Could you check a few things on this model? Use its own coordinates, in mm. Face numbers are marked on the shaded views. A direction names the side the tool comes from. Give positions to 0.01 mm unless a question says otherwise; leave off trailing zeros. Loops run counter-clockwise (first coordinate to the right, second up) from the corner with the lowest first, then second, coordinate; pieces in that order, holes last.
1. Thinking about a two-plate mould opening in Z: for the marked faces 1, 2 and 3, which applies, +Z half, -Z half, draft (parallel to the pull), parting line (faces both ways), or undercut?
2. For the marked faces 4 and 5, which set-ups out of +Z, -Z, +X, -X, +Y, -Y let a thin tool reach every point of the face, with its end or its side?
3. Imagine slicing it at D-D (x = -113). List the corners of the cut face in (y, z) for me, plus the area to 3 significant figures.
4. Imagine slicing it at A-A (y = 39.5). List the corners of the cut face in (x, z) for me, plus the area to 3 significant figures.
5. I need wall thicknesses on line 1 along Z through (x, y) = (-99.5, 18); line 2 along X through (y, z) = (8, 0); line 3 along Z through (x, y) = (-61.5, 8.25). Which ranges of each line are inside material? Lowest first, please.
6. Imagine slicing it at B-B (x = -39). List the corners of the cut face in (y, z) for me, plus the area to 3 significant figures.
7. Imagine slicing it at C-C (y = 5). Count the separate pieces of the cut face and the enclosed holes in it, plus the area to 3 significant figures.
8. For P1, Ø1.5, axis at x = -52.5, z = 15, coming from the +Y side; P2, Ø3.5, axis at y = 18.5, z = -28, coming from the +X side; P3, Ø11, axis at x = -90, z = 0, coming from the -Y side (3 decimals); P4, Ø4, axis at y = 21, z = -11, coming from the -X side, each with a flat end and sliding along its axis, tell me the tip position at first contact or that it passes through.
```python
from build123d import *

# Parameters (mm, degrees)
BOSS_EXTRUDE1_DEPTH        = 10
BOSS_EXTRUDE2_DEPTH        = 32
CUT_EXTRUDE1_REACH         = 207
SKETCH3_R                  = 2.55
SKETCH3_W                  = 40
SKETCH3_H                  = 25
FILLET1_R                  = 1.2
SKETCH4_R                  = 7
SKETCH4_R_2                = 17.5
CUT_EXTRUDE2_DEPTH         = 11
SKETCH5_R                  = 21
CUT_EXTRUDE3_DEPTH         = 7
SKETCH6_R                  = 14
SKETCH6_R_2                = 11
BOSS_EXTRUDE3_DEPTH        = 6
CUT_EXTRUDE4_DEPTH         = 11
SKETCH8_R                  = 11
CUT_EXTRUDE5_DEPTH         = 7
SKETCH9_R                  = 2.1
SKETCH9_R_2                = 2.5
SKETCH9_R_3                = 1.6
CUT_EXTRUDE6_DEPTH         = 11
BOSS_EXTRUDE4_DEPTH        = 7
CHAMFER1_SIZE              = 2
LPATTERN1_COUNT            = 3
LPATTERN1_PITCH            = 40
CHAMFER1_OF_LPATTERN1_SIZE = 2
CUT_EXTRUDE7_DEPTH         = 12
LPATTERN2_COUNT            = 3
LPATTERN2_PITCH            = 64
MIRROR1_COPY_1_DEPTH       = 12
MIRROR1_COPY_2_DEPTH       = 12
CUT_REVOLVE1_ANGLE         = 20
SKETCH13_R                 = 11
CUT_EXTRUDE8_DEPTH         = 1


with BuildPart() as part:
    # Sketch1 → Boss-Extrude1 (new body)
    with BuildSketch(Plane(origin=(0, 0, 0), x_dir=(1, 0, 0), z_dir=(0, 1, 0))):
        with BuildLine():
            Line((0, 39), (-166, 39))
            Line((-166, 39), (-166, -39))
            Line((-166, -39), (0, -39))
            ThreePointArc((0, -39), (39, 0), (0, 39))
        make_face()
    extrude(amount=BOSS_EXTRUDE1_DEPTH)

    # Sketch2 → Boss-Extrude2 (add)
    with BuildSketch(Plane(origin=(0, 10, 0), x_dir=(1, 0, 0), z_dir=(0, 1, 0))):
        with BuildLine():
            Line((0, 39), (-166, 39))
            Line((-166, 39), (-166, -39))
            Line((-166, -39), (0, -39))
            ThreePointArc((0, -39), (39, 0), (0, 39))
        make_face()
        with BuildLine():
            Line((0, 35), (-158, 35))
            Line((-158, 35), (-158, -35))
            Line((-158, -35), (0, -35))
            ThreePointArc((0, -35), (35, 0), (0, 35))
        make_face(mode=Mode.SUBTRACT)
    extrude(amount=BOSS_EXTRUDE2_DEPTH)

    # Sketch3 → Cut-Extrude1 (cut, up to next)
    with BuildSketch(Plane.ZY.offset(166), mode=Mode.PRIVATE) as cut_extrude1_sk1:
        with Locations((-25.5, 34.5)):
            Circle(SKETCH3_R)
    cut_extrude1_tool1 = extrude(cut_extrude1_sk1.sketch, amount=-CUT_EXTRUDE1_REACH, mode=Mode.PRIVATE) & part.part
    add(cut_extrude1_tool1.solids().sort_by_distance((-166, 34.5, -25.5))[0], mode=Mode.SUBTRACT)
    # Sketch3 → Cut-Extrude1 (cut, up to next)
    with BuildSketch(Plane.ZY.offset(166), mode=Mode.PRIVATE) as cut_extrude1_sk2:
        with Locations((-25.5, 16.5)):
            Circle(SKETCH3_R)
    cut_extrude1_tool2 = extrude(cut_extrude1_sk2.sketch, amount=-CUT_EXTRUDE1_REACH, mode=Mode.PRIVATE) & part.part
    add(cut_extrude1_tool2.solids().sort_by_distance((-166, 16.5, -25.5))[0], mode=Mode.SUBTRACT)
    # Sketch3 → Cut-Extrude1 (cut, up to next)
    with BuildSketch(Plane.ZY.offset(166), mode=Mode.PRIVATE) as cut_extrude1_sk3:
        with Locations((25.5, 16.5)):
            Circle(SKETCH3_R)
    cut_extrude1_tool3 = extrude(cut_extrude1_sk3.sketch, amount=-CUT_EXTRUDE1_REACH, mode=Mode.PRIVATE) & part.part
    add(cut_extrude1_tool3.solids().sort_by_distance((-166, 16.5, 25.5))[0], mode=Mode.SUBTRACT)
    # Sketch3 → Cut-Extrude1 (cut, up to next)
    with BuildSketch(Plane.ZY.offset(166), mode=Mode.PRIVATE) as cut_extrude1_sk4:
        with Locations((25.5, 34.5)):
            Circle(SKETCH3_R)
    cut_extrude1_tool4 = extrude(cut_extrude1_sk4.sketch, amount=-CUT_EXTRUDE1_REACH, mode=Mode.PRIVATE) & part.part
    add(cut_extrude1_tool4.solids().sort_by_distance((-166, 34.5, 25.5))[0], mode=Mode.SUBTRACT)
    # Sketch3 → Cut-Extrude1 (cut, up to next)
    with BuildSketch(Plane.ZY.offset(166), mode=Mode.PRIVATE) as cut_extrude1_sk5:
        with Locations((0, 24.5)):
            Rectangle(SKETCH3_W, SKETCH3_H)
    cut_extrude1_tool5 = extrude(cut_extrude1_sk5.sketch, amount=-CUT_EXTRUDE1_REACH, mode=Mode.PRIVATE) & part.part
    add(cut_extrude1_tool5.solids().sort_by_distance((-166, 24.5, 0))[0], mode=Mode.SUBTRACT)

    # Fillet1
    fillet1_edges = [part.edges().sort_by_distance(p)[0] for p in [
        (-162, 37, -20),
        (-162, 12, -20),
        (-162, 12, 20),
        (-162, 37, 20),
    ]]
    fillet(fillet1_edges, radius=FILLET1_R)

    # Sketch4 → Cut-Extrude2 (cut, through all)
    with BuildSketch(Plane(origin=(0, 10, 0), x_dir=(1, 0, 0), z_dir=(0, 1, 0))):
        with Locations((-90, 0)):
            Circle(SKETCH4_R)
        Circle(SKETCH4_R_2)
    extrude(amount=-CUT_EXTRUDE2_DEPTH, mode=Mode.SUBTRACT)

    # Sketch5 → Cut-Extrude3 (cut)
    with BuildSketch(Plane(origin=(0, 10, 0), x_dir=(1, 0, 0), z_dir=(0, 1, 0))):
        Circle(SKETCH5_R)
    extrude(amount=-CUT_EXTRUDE3_DEPTH, mode=Mode.SUBTRACT)

    # Sketch6 → Boss-Extrude3 (add)
    with BuildSketch(Plane(origin=(0, 10, 0), x_dir=(1, 0, 0), z_dir=(0, 1, 0))):
        with Locations((-90, 0)):
            Circle(SKETCH6_R)
        with Locations((-90, 0)):
            Circle(SKETCH6_R_2, mode=Mode.SUBTRACT)
    extrude(amount=BOSS_EXTRUDE3_DEPTH)

    # Sketch7 → Cut-Extrude4 (cut, through all)
    with BuildSketch(Plane(origin=(0, 10, 0), x_dir=(1, 0, 0), z_dir=(0, 1, 0))):
        with BuildLine():
            Line((-132.5, 23), (-132.5, 13))
            ThreePointArc((-132.5, 13), (-135, 10.5), (-137.5, 13))
            Line((-137.5, 13), (-137.5, 23))
            ThreePointArc((-137.5, 23), (-135, 25.5), (-132.5, 23))
        make_face()
        with BuildLine():
            Line((-132.5, -13), (-132.5, -23))
            ThreePointArc((-132.5, -23), (-135, -25.5), (-137.5, -23))
            Line((-137.5, -23), (-137.5, -13))
            ThreePointArc((-137.5, -13), (-135, -10.5), (-132.5, -13))
        make_face()
        with BuildLine():
            Line((-47.5, 25), (-47.5, 13))
            ThreePointArc((-47.5, 13), (-50, 10.5), (-52.5, 13))
            Line((-52.5, 13), (-52.5, 25))
            ThreePointArc((-52.5, 25), (-50, 27.5), (-47.5, 25))
        make_face()
        with BuildLine():
            Line((-47.5, -21), (-47.5, -25))
            ThreePointArc((-47.5, -25), (-50, -27.5), (-52.5, -25))
            Line((-52.5, -25), (-52.5, -21))
            ThreePointArc((-52.5, -21), (-50, -18.5), (-47.5, -21))
        make_face()
    extrude(amount=-CUT_EXTRUDE4_DEPTH, mode=Mode.SUBTRACT)

    # Sketch8 → Cut-Extrude5 (cut)
    with BuildSketch(Plane.XZ):
        with Locations((-90, 0)):
            Circle(SKETCH8_R)
    extrude(amount=-CUT_EXTRUDE5_DEPTH, mode=Mode.SUBTRACT)

    # Sketch9 → Cut-Extrude6 (cut, through all)
    with BuildSketch(Plane(origin=(0, 10, 0), x_dir=(1, 0, 0), z_dir=(0, 1, 0))):
        with Locations((-39, 27)):
            Circle(SKETCH9_R)
        with Locations((-61.5, 10.809700388)):
            Circle(SKETCH9_R_2)
        with Locations((-58, -9.459979846)):
            Circle(SKETCH9_R_3)
        with Locations((-49.611997868, -5)):
            Circle(SKETCH9_R_3)
    extrude(amount=-CUT_EXTRUDE6_DEPTH, mode=Mode.SUBTRACT)

    # Sketch10 → Boss-Extrude4 (add)
    with BuildSketch(Plane(origin=(-145, 0, 0), x_dir=(0, 0, -1), z_dir=(1, 0, 0))):
        Polygon((27, 10), (31, 10), (31, 19), (32, 20), (32, 21), (31, 22), (27, 22), align=None)
    boss_extrude4 = extrude(amount=BOSS_EXTRUDE4_DEPTH)

    # Chamfer1
    chamfer1_edges = [part.edges().sort_by_distance(p)[0] for p in [
        (-141.5, 10, -27),
    ]]
    chamfer(chamfer1_edges, length=CHAMFER1_SIZE)

    # LPattern1: Boss-Extrude4 ×3
    with Locations(*[(i * LPATTERN1_PITCH, 0, 0) for i in range(1, LPATTERN1_COUNT)]):
        add(boss_extrude4)

    # Chamfer1 of LPattern1
    chamfer1_of_lpattern1_edges = [part.edges().sort_by_distance(p)[0] for p in [
        (-101.5, 10, -27),
        (-61.5, 10, -27),
    ]]
    chamfer(chamfer1_of_lpattern1_edges, length=CHAMFER1_OF_LPATTERN1_SIZE)

    # Sketch11 → Cut-Extrude7 (cut)
    with BuildSketch(Plane.ZY.offset(142)):
        Polygon((-35, 34.6), (-35, 36.9), (-35.55, 36.35), (-35.55, 35.15), align=None)
    cut_extrude7 = extrude(amount=-CUT_EXTRUDE7_DEPTH, mode=Mode.SUBTRACT)

    # LPattern2: Cut-Extrude7 ×3
    with Locations(*[(i * LPATTERN2_PITCH, 0, 0) for i in range(1, LPATTERN2_COUNT)]):
        add(cut_extrude7, mode=Mode.SUBTRACT)

    # Mirror1: Cut-Extrude7 across plane
    add(cut_extrude7.mirror(Plane.XY), mode=Mode.SUBTRACT)

    # Mirror1 copy 1 sketch → Mirror1 copy 1 (cut)
    with BuildSketch(Plane(origin=(-78, 0, 0), x_dir=(0, 0, -1), z_dir=(-1, 0, 0))):
        Polygon((-35, -34.6), (-35, -36.9), (-35.55, -36.35), (-35.55, -35.15), align=None)
    extrude(amount=-MIRROR1_COPY_1_DEPTH, mode=Mode.SUBTRACT)

    # Mirror1 copy 2 sketch → Mirror1 copy 2 (cut)
    with BuildSketch(Plane(origin=(-14, 0, 0), x_dir=(0, 0, -1), z_dir=(-1, 0, 0))):
        Polygon((-35, -34.6), (-35, -36.9), (-35.55, -36.35), (-35.55, -35.15), align=None)
    extrude(amount=-MIRROR1_COPY_2_DEPTH, mode=Mode.SUBTRACT)

    # Sketch12 → Cut-Revolve1 (revolve, symmetric, cut)
    with BuildSketch(Plane.XY) as cut_revolve1_sk:
        Polygon((35.55, 36.35), (35, 36.9), (35, 34.6), (35.55, 35.15), align=None)
    revolve(axis=Axis((0, 42, 0), (0, -1, 0)), revolution_arc=CUT_REVOLVE1_ANGLE / 2, mode=Mode.SUBTRACT)
    revolve(cut_revolve1_sk.sketch, axis=Axis((0, 42, 0), (0, 1, 0)), revolution_arc=CUT_REVOLVE1_ANGLE / 2, mode=Mode.SUBTRACT)

    # Sketch13 → Cut-Extrude8 (cut)
    with BuildSketch(Plane(origin=(0, 10, 0), x_dir=(1, 0, 0), z_dir=(0, 1, 0))):
        with Locations((-90, 0)):
            Circle(SKETCH13_R)
    extrude(amount=-CUT_EXTRUDE8_DEPTH, mode=Mode.SUBTRACT)


solid = part.part
```
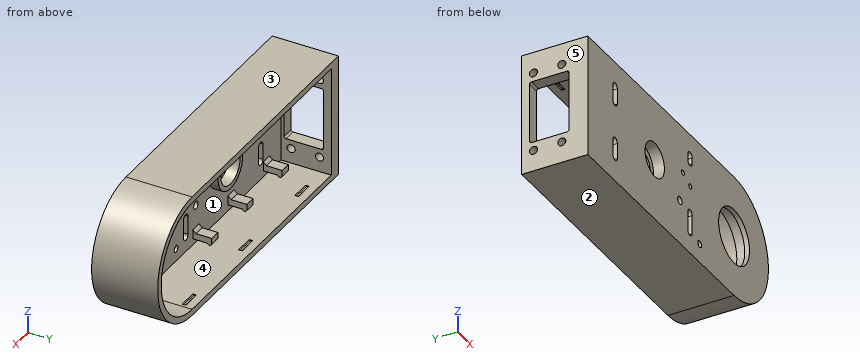
Derived:
1. face 1: undercut
1. face 2: -Z half
1. face 3: +Z half
2. face 4: +Y
2. face 5: +Z, -Z, -X, +Y, -Y
3. outline: (0, -39) - (42, -39) - (42, -35) - (10, -35) - (10, 35) - (42, 35) - (42, 39) - (0, 39) - close
3. area: 1,040 mm2
4. outline: (-166, -39) - (0, -39) arc R39 ccw to (0, 39) - (-166, 39) - close; hole (-158, -35) - (0, -35) arc R35 ccw to (0, 35) - (-158, 35) - close
4. area: 2,350 mm2
5. line 1: z = -39 to -35, -31 to -27, 35 to 39
5. line 2: x = -166 to -97, -83 to -21, 21 to 39
5. line 3: z = -39 to -13.31, -8.31 to 39
6. outline: (0, -39) - (42, -39) - (42, -35) - (10, -35) - (10, -29.1) - (0, -29.1) - close; (0, -24.9) - (10, -24.9) - (10, 35) - (42, 35) - (42, 39) - (0, 39) - close
6. area: 994 mm2
7. separate pieces: 1
7. enclosed holes: 10
7. area: 13,300 mm2
8. P1: stops at y = 10
8. P2: stops at x = 28.84
8. P3: passes through
8. P4: stops at x = 32.5
